Here's how the part is built. I have some questions about the finished solid (model axes, mm). Round coordinates to 2 decimals unless told otherwise and drop trailing zeros. Write each loop counter-clockwise with the first axis right and the second up, starting at its lowest first coordinate (ties: lowest second). Pieces come first, ordered by that corner, then holes. Notation, with made-up numbers: M 60,77 L 92,77 A20 ccw 92,108 Z; hole C 56,-23.75 d4. An arc over 180 degrees is marked long. Use one line per item in the form item = value. Start each with the question number.
Q1. I need wall thicknesses on line 1 along Y through (x, z) = (2.75, 0); line 2 along Z through (x, y) = (149.5, 0.15); line 3 along Y through (x, z) = (73, -0.35). Which ranges of each line are inside material? Lowest first, please. Write a range as from..to.
Q2. I want a section at A-A on x = 200. List the corners of the cut face in (y, z) for me, and give its area (3 significant figures).
Q3. I'm going to push flat-ended pins straight in: pin 1 Ø2 at (x, z) = (64, 2) entering from +Y; pin 2 Ø2 at (y, z) = (0, 0) entering from +X. Where does each tip first touch, or does it pass through?
```python
from build123d import *

# Parameters (mm, degrees)
SKETCH1_R                       = 3
BOSS_EXTRUDE1_DEPTH             = 300
M4_TAPPED_HOLE2_D               = 3.3
M4_TAPPED_HOLE2_DEPTH           = 10.1
M4_TAPPED_HOLE2_TIP             = 0.991420021
M4_TAPPED_HOLE2_ON_FACE_2_D     = 3.3
M4_TAPPED_HOLE2_ON_FACE_2_DEPTH = 10.1
M4_TAPPED_HOLE2_ON_FACE_2_TIP   = 0.991420021


with BuildPart() as part:
    # Sketch1 → Boss-Extrude1 (new body)
    with BuildSketch(Plane(origin=(0, 0, 0), x_dir=(0, 0, -1), z_dir=(1, 0, 0))):
        Circle(SKETCH1_R)
    extrude(amount=BOSS_EXTRUDE1_DEPTH)

    # M4 Tapped Hole2
    with Locations(Plane(origin=(0, 0, 0), x_dir=(0, 0, -1), z_dir=(-1, 0, 0))):
        with Locations((0, 0)):
            Hole(M4_TAPPED_HOLE2_D / 2, depth=M4_TAPPED_HOLE2_DEPTH)
            with Locations((0, 0, -(M4_TAPPED_HOLE2_DEPTH + M4_TAPPED_HOLE2_TIP / 2))):  # 118° drill point
                Cone(0, M4_TAPPED_HOLE2_D / 2, M4_TAPPED_HOLE2_TIP, mode=Mode.SUBTRACT)

    # M4 Tapped Hole2 on face 2
    with Locations(Plane(origin=(300, 0, 0), x_dir=(0, 0, 1), z_dir=(1, 0, 0))):
        with Locations((0, 0)):
            Hole(M4_TAPPED_HOLE2_ON_FACE_2_D / 2, depth=M4_TAPPED_HOLE2_ON_FACE_2_DEPTH)
            with Locations((0, 0, -(M4_TAPPED_HOLE2_ON_FACE_2_DEPTH + M4_TAPPED_HOLE2_ON_FACE_2_TIP / 2))):  # 118° drill point
                Cone(0, M4_TAPPED_HOLE2_ON_FACE_2_D / 2, M4_TAPPED_HOLE2_ON_FACE_2_TIP, mode=Mode.SUBTRACT)


solid = part.part
```
Reported:
q1.line_1 = -3..-1.65, 1.65..3
q1.line_2 = -3..3
q1.line_3 = -2.98..2.98
q2.outline = C 0,0 d6
q2.area = 28.3 mm^2
q3.pin_1 = 2.83
q3.pin_2 = 289.51
